Autodesk Inventor part; units mm, degrees
ref_plane "YZ Plane" through (0, 0, 0) normal (1, 0, 0) x (0, 1, 0)
ref_plane "XZ Plane" through (0, 0, 0) normal (0, 1, 0) x (-1, 0, 0)
ref_plane "XY Plane" through (0, 0, 0) normal (0, 0, 1) x (1, 0, 0)
sketch "Sketch1" plane through (0, 0, 0) normal (0, 1, 0) x (-1, 0, 0)
  line L0 (-14.5799, 0) -> (14.5799, 0)
  line L1 (7, 5) -> (-7, 5)
  line L2 (-7, 5) -> (-7, -5)
  line L3 (-7, -5) -> (7, -5)
  line L4 (7, -5) -> (7, 5)
  line L5 (8, 7.5) -> (-8, 7.5)
  line L6 (-10, 5.5) -> (-10, -5.5)
  line L7 (-8, -7.5) -> (8, -7.5)
  line L8 (10, -5.5) -> (10, 5.5)
  line L9 (0, -11.0799) -> (0, 11.0799)
  arc A0 (10, 5.5) -> (8, 7.5) centre (8, 5.5) ccw
  arc A1 (8, -7.5) -> (10, -5.5) centre (8, -5.5) ccw
  arc A2 (-10, -5.5) -> (-8, -7.5) centre (-8, -5.5) ccw
  arc A3 (-8, 7.5) -> (-10, 5.5) centre (-8, 5.5) ccw
  line L10 (-4, 2.5) -> (4, 2.5)
  line L11 (4, 2.5) -> (4, -2.5)
  line L12 (4, -2.5) -> (-4, -2.5)
  line L13 (-4, -2.5) -> (-4, 2.5)
  point P0 (0, 0)
  point P1 (10, 7.5)
  point P2 (10, -7.5)
  dimension "d0" = 10
  dimension "d1" = 15
  dimension "d2" = 14
  dimension "d3" = 20
  dimension "d4" = 2
  dimension "d9" = 5
  dimension "d10" = 8
extrude "Extrusion1" add sketch "Sketch1" against normal blind 4 contours L6 A3 L5 L9 L1 L2 L0 | L0 L2 L3 L9 L7 A2 L6 | L9 L5 A0 L8 L0 L4 L1 | L3 L4 L0 L8 A1 L7 L9
extrude "Extrusion3" add sketch "Sketch1" against normal blind 8 contours L13 L10 L9 L0 | L0 L9 L12 L13 | L9 L10 L11 L0 | L0 L11 L12 L9
extrude "Extrusion4" add sketch "Sketch1" against normal blind 9 contours L2 L1 L9 L10 L13 L0 | L0 L13 L12 L9 L3 L2 | L1 L4 L0 L11 L10 L9 | L9 L12 L11 L0 L4 L3
properties part number "slab"
Could you check a few things on this model? Use its own coordinates, in mm. A direction names the side the tool comes from. Coordinates: 2 decimals unless noted, no trailing zeros. Write each loop counter-clockwise with the first axis right and the second up, starting at its lowest first coordinate (ties: lowest second). Pieces come first, ordered by that corner, then holes. Notation, with made-up numbers: (38, -9) - (45, -9) arc R11 cw to (45, -5) - close; hole circle Ø9 at (-30.5, 10). An arc over 180 degrees is marked (long way). Write item = value, one per line.
1) Suppose I cut it at C-C on y = -5.5. Please give me the cut outline in (x, z).
Result set:
outline = (-7, -5) - (7, -5) - (7, 5) - (-7, 5) - close
2) For faces 5 (the flat face through (4, -8.5, 0)), 6 (the flat face through (7, -6, 0)), 7 (the flat face through (0, -6, 5)), which set-ups out of +Z, -Z, +X, -X, +Y, -Y let a thin tool reach every point of the face, with its end or its side?
Result set:
face_5 = -Y
face_6 = +Z, -Z, +X, -Y
face_7 = +Z, +X, -X, -Y
3) Please list where these lines run through material, in increasing order: line 1 (Y direction, x = -2.25, z = -0.5); line 2 (Z direction, x = 2.5, y = -7.5); line 3 (Y direction, x = 0.5, z = 7). Write a range as [from, to].
Result set:
line_1 = [-8, 0]
line_2 = [-5, 5]
line_3 = [-4, 0]
4) We'd pull the mould along Z, two halves only. Please class faces 1 (the flat face through (-0.1, -8.5, -2.5)), 2 (the flat face through (0, -8, 0)), 3 (the cylindrical face through (-9.4, -1.97, -6.93)), 4 (the flat face through (0, -2, 7.5)): +Z half, -Z half, draft (parallel to the pull), parting line (faces both ways), or undercut.
Result set:
face_1 = undercut
face_2 = undercut
face_3 = -Z half
face_4 = +Z half
5) Suppose I cut it at B-B on x = 0.25. Please give me the cut outline in (y, z).
Result set:
outline = (-9, -5) - (-4, -5) - (-4, -7.5) - (0, -7.5) - (0, 7.5) - (-4, 7.5) - (-4, 5) - (-9, 5) - (-9, 2.5) - (-8, 2.5) - (-8, -2.5) - (-9, -2.5) - close
6) Will these pins go through, and if not, where does the flat tip stop? pin 1 Ø1.5 at (x, z) = (-2, -1) entering from -Y; pin 2 Ø2.5 at (x, y) = (3.5, -6) entering from -Z; pin 3 Ø1.1 at (y, z) = (-8.5, 1) entering from -X.
Result set:
pin_1 = -8
pin_2 = -5
pin_3 = -7
7) Suppose I cut it at A-A on z = -4.75. Please give me the cut outline in (x, y).
Result set:
outline = (-10, -4) - (-7, -4) - (-7, -9) - (7, -9) - (7, -4) - (10, -4) - (10, 0) - (-10, 0) - close
8) Suppose I cut it at D-D on x = -6. Please give me the cut outline in (y, z).
Result set:
outline = (-9, -5) - (-4, -5) - (-4, -7.5) - (0, -7.5) - (0, 7.5) - (-4, 7.5) - (-4, 5) - (-9, 5) - close
